The listing builds one solid part. Answer for the finished solid, in the listing's coordinates (mm). Give positions to 0.01 mm unless a question says otherwise; leave off trailing zeros. Loops run counter-clockwise (first coordinate to the right, second up) from the corner with the lowest first, then second, coordinate; pieces in that order, holes last. Notation, with made-up numbers: M 31,61 L 70,61 A14 ccw 70,65 Z; hole C 81,3 d10. An arc over 180 degrees is marked long. Use one line per item in the form item = value. Start each with the question number.
1. Straight lines are drawn through the part: line 1 (Y direction, x = -69.5, z = 1.35); line 2 (Y direction, x = 78.5, z = 0.8); line 3 (X direction, y = 65, z = 0.4). For each, find the intervals that lie inside material, in ascending order. Write a range as from..to.
2. The part is cut by section A-A (z = 0.4). Give the number of separate pieces and of enclosed holes in the cut face, and give its area (3 significant figures).
3. The part is cut by section B-B (y = -79.5). Write down the section's boundary in (x, z), and give its area (3 significant figures).
4. This flat-tipped pin is pushed along its axis until it touches: pin 1 Ø8 at (x, y) = (-78.5, 153) entering from -Z. Where does it stop, or does it pass through?
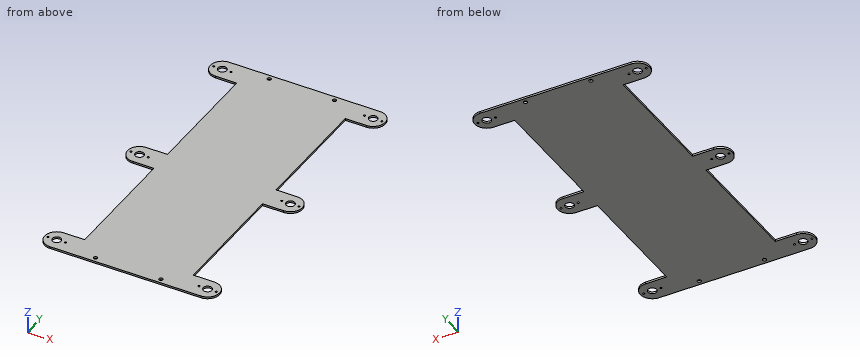
from build123d import *

# Parameters (mm, degrees)
ESQUISSE1_R        = 4.5
ESQUISSE1_R_2      = 2
ESQUISSE1_R_3      = 1
BOSS_EXTRU_1_DEPTH = 2


with BuildPart() as part:
    # Esquisse1 → Boss.-Extru.1 (new body)
    with BuildSketch(Plane.XY):
        with BuildLine():
            Line((-78.5, 165.5), (78.5, 165.5))
            ThreePointArc((78.5, 165.5), (91, 153), (78.5, 140.5))
            Line((78.5, 140.5), (56.5, 140.5))
            Line((56.5, 140.5), (56.5, 12.5))
            Line((56.5, 12.5), (78.5, 12.5))
            ThreePointArc((78.5, 12.5), (91, 0), (78.5, -12.5))
            Line((78.5, -12.5), (56.5, -12.5))
            Line((56.5, -12.5), (56.5, -140.5))
            Line((56.5, -140.5), (78.5, -140.5))
            ThreePointArc((78.5, -140.5), (91, -153), (78.5, -165.5))
            Line((78.5, -165.5), (-78.5, -165.5))
            ThreePointArc((-78.5, -165.5), (-91, -153), (-78.5, -140.5))
            Line((-78.5, -140.5), (-56.5, -140.5))
            Line((-56.5, -140.5), (-56.5, -12.5))
            Line((-56.5, -12.5), (-78.5, -12.5))
            ThreePointArc((-78.5, -12.5), (-91, 0), (-78.5, 12.5))
            Line((-78.5, 12.5), (-56.5, 12.5))
            Line((-56.5, 12.5), (-56.5, 140.5))
            Line((-56.5, 140.5), (-78.5, 140.5))
            ThreePointArc((-78.5, 140.5), (-91, 153), (-78.5, 165.5))
        make_face()
        with Locations((78.5, 153)):
            Circle(ESQUISSE1_R, mode=Mode.SUBTRACT)
        with Locations((78.5, 0)):
            Circle(ESQUISSE1_R, mode=Mode.SUBTRACT)
        with Locations((78.5, -153)):
            Circle(ESQUISSE1_R, mode=Mode.SUBTRACT)
        with Locations((34, 160.5)):
            Circle(ESQUISSE1_R_2, mode=Mode.SUBTRACT)
        with Locations((69.5, 153)):
            Circle(ESQUISSE1_R_3, mode=Mode.SUBTRACT)
        with Locations(Location((87.5, 153, 0), (0, 0, 180))):
            Circle(ESQUISSE1_R_3, mode=Mode.SUBTRACT)
        with Locations((69.5, 0)):
            Circle(ESQUISSE1_R_3, mode=Mode.SUBTRACT)
        with Locations((69.5, -153)):
            Circle(ESQUISSE1_R_3, mode=Mode.SUBTRACT)
        with Locations(Location((87.5, 0, 0), (0, 0, 180))):
            Circle(ESQUISSE1_R_3, mode=Mode.SUBTRACT)
        with Locations(Location((87.5, -153, 0), (0, 0, 180))):
            Circle(ESQUISSE1_R_3, mode=Mode.SUBTRACT)
        with Locations(Location((34, -160.5, 0), (0, 0, 180))):
            Circle(ESQUISSE1_R_2, mode=Mode.SUBTRACT)
        with Locations(Location((-78.5, 153, 0), (0, 0, 180))):
            Circle(ESQUISSE1_R, mode=Mode.SUBTRACT)
        with Locations((-87.5, 153)):
            Circle(ESQUISSE1_R_3, mode=Mode.SUBTRACT)
        with Locations(Location((-69.5, 153, 0), (0, 0, 180))):
            Circle(ESQUISSE1_R_3, mode=Mode.SUBTRACT)
        with Locations(Location((-34, 160.5, 0), (0, 0, 180))):
            Circle(ESQUISSE1_R_2, mode=Mode.SUBTRACT)
        with Locations((-87.5, 0)):
            Circle(ESQUISSE1_R_3, mode=Mode.SUBTRACT)
        with Locations(Location((-78.5, 0, 0), (0, 0, 180))):
            Circle(ESQUISSE1_R, mode=Mode.SUBTRACT)
        with Locations(Location((-69.5, 0, 0), (0, 0, 180))):
            Circle(ESQUISSE1_R_3, mode=Mode.SUBTRACT)
        with Locations((-87.5, -153)):
            Circle(ESQUISSE1_R_3, mode=Mode.SUBTRACT)
        with Locations(Location((-69.5, -153, 0), (0, 0, 180))):
            Circle(ESQUISSE1_R_3, mode=Mode.SUBTRACT)
        with Locations(Location((-78.5, -153, 0), (0, 0, 180))):
            Circle(ESQUISSE1_R, mode=Mode.SUBTRACT)
        with Locations((-34, -160.5)):
            Circle(ESQUISSE1_R_2, mode=Mode.SUBTRACT)
    extrude(amount=BOSS_EXTRU_1_DEPTH)


solid = part.part
Derived:
q1.line_1 = -165.5..-154, -152..-140.5, -12.5..-1, 1..12.5, 140.5..152, 154..165.5
q1.line_2 = -165.5..-157.5, -148.5..-140.5, -12.5..-4.5, 4.5..12.5, 140.5..148.5, 157.5..165.5
q1.line_3 = -56.5..56.5
q2.separate_pieces = 1
q2.enclosed_holes = 22
q2.area = 41,700 mm2
q3.outline = M -56.5,0 L 56.5,0 L 56.5,2 L -56.5,2 Z
q3.area = 226 mm2
q4.pin_1 = through
